```python
from build123d import *

# Parameters (mm, degrees)
CHAFL_N4_SIZE              = 0.2
CHAFL_N5_SIZE              = 0.25
CHAFL_N5_SIZE2             = 0.433012702
CORTAR_EXTRUIR2_DEPTH      = 17.552945357
CORTAR_EXTRUIR2_DEPTH_BACK = 17.552945357
CROQUIS4_W                 = 0.8
CROQUIS4_H                 = 6


with BuildPart() as part:
    # Croquis3 → Revolución1 (revolve)
    with BuildSketch(Plane.XY, mode=Mode.PRIVATE) as revoluci_n1_sk:
        Polygon((-1.6, 0), (-1.6, 16), (-2.4, 16), (-2.4, 13), (-3, 13), (-3, 7.5), (-2.1, 7.5), (-2.1, 5.5), (-3, 5.5), (-3, 0), align=None)
    revolve(revoluci_n1_sk.sketch.rotate(Axis((0, 0, 0), (0, 1, 0)), 270), axis=Axis((0, 0, 0), (0, 1, 0)))

    # Chaflán4
    chafl_n4_edges = [part.edges().sort_by_distance(p)[0] for p in [
        (0, 16, 2.4),
        (0, 0, 3),
    ]]
    chamfer(chafl_n4_edges, length=CHAFL_N4_SIZE)

    # Chaflán5
    chafl_n5_edges = [part.edges().sort_by_distance(p)[0] for p in [
        (0, 16, 1.6),
    ]]
    chafl_n5_side = [part.faces().sort_by_distance(p)[0] for p in [
        (0, 16, 2.137774603),
    ]]
    chamfer(chafl_n5_edges, length=CHAFL_N5_SIZE, length2=CHAFL_N5_SIZE2, reference=chafl_n5_side[0])

    # Croquis4 → Cortar-Extruir2 (cut, two sides: drawn at the far end of the back side and taken through both)
    with BuildSketch(Plane.XY.offset(-CORTAR_EXTRUIR2_DEPTH_BACK)):
        with Locations((-2.6, 6.5)):
            Rectangle(CROQUIS4_W, CROQUIS4_H)
        with Locations((2.6, 6.5)):
            Rectangle(CROQUIS4_W, CROQUIS4_H)
    extrude(amount=CORTAR_EXTRUIR2_DEPTH + CORTAR_EXTRUIR2_DEPTH_BACK, mode=Mode.SUBTRACT)


solid = part.part
```
Here's how the part is built. I have some questions about the finished solid (model axes, mm). A direction names the side the tool comes from. Give positions to 0.01 mm unless a question says otherwise; leave off trailing zeros. Write each loop counter-clockwise with the first axis right and the second up, starting at its lowest first coordinate (ties: lowest second). Pieces come first, ordered by that corner, then holes. Notation, with made-up numbers: M 62.25,-33 L 91.25,-33 A22 cw 91.25,-18 Z; hole C 23.25,-30.75 d6. An arc over 180 degrees is marked long. Put each result on its own line as item: value. Start each with the question number.
Item 1: I need wall thicknesses on L1, parallel to Z at x = -0.1, y = 8; L2, parallel to X at y = 8, z = 0. Which ranges of each line are inside material? Lowest first, please. Write a range as from..to.
Item 2: Will these pins go through, and if not, where does the flat tip stop? pin 1 (2 mm diameter, centred on y = 8, z = 0, fed in from +X); pin 2 (1.3 mm diameter, centred on x = 0, z = 0.5, fed in from -Y).
Item 3: On a 3-axis mill with a long thin cutter (end or side, diameter ignored), from which of +Z, -Z, +X, -X, +Y, -Y can I reach the whole of each face in a straight line? I mean faces 4 (the flat face through (2.5, 3.5, 0)), 5 (the cylindrical face through (-0.631, 6.486, -2.003)), 6 (the flat face through (-2.2, 8, 0)). Say none if no direction works.
Item 4: If we section it at C-C, the plane y = 4.75: Write out the boundary of the cut face in (x, z), then the cut area to 3 significant figures.
Item 5: If we section it at B-B, the plane x = 0: Write out the boundary of the cut face in (y, z), then the cut area to 3 significant figures.
Item 6: Thinking about a two-plate mould opening in Z: for faces 1 (the flat face through (-2.2, 4, 0)), 2 (the cylindrical face through (0.97, 7.89, 1.27)), 3 (the cylindrical face through (-2.024, 14.38, -1.29)), which applies, +Z half, -Z half, draft (parallel to the pull), parting line (faces both ways), or undercut?
Item 7: If we section it at D-D, the plane y = 14.5: Write out the boundary of the cut face in (x, z), then the cut area to 3 significant figures.
Values:
1. L1: -3..-1.6, 1.6..3
1. L2: -2.2..-1.6, 1.6..2.2
2. pin 1: x = 2.2
2. pin 2: through
3. face 4: +Z, -Z, +X
3. face 5: none
3. face 6: +Z, -Z, -X
4. outline: M -2.2,-2.04 A3 ccw 2.2,-2.04 L 2.2,2.04 A3 ccw -2.2,2.04 Z; hole C 0,0 d3.2
4. area: 15.7 mm²
5. outline: M 0,-2.8 L 0.2,-3 L 5.5,-3 L 5.5,-2.1 L 7.5,-2.1 L 7.5,-3 L 13,-3 L 13,-2.4 L 15.8,-2.4 L 16,-2.2 L 16,-1.85 L 15.57,-1.6 L 0,-1.6 Z; M 0,1.6 L 15.57,1.6 L 16,1.85 L 16,2.2 L 15.8,2.4 L 13,2.4 L 13,3 L 7.5,3 L 7.5,2.1 L 5.5,2.1 L 5.5,3 L 0.2,3 L 0,2.8 Z
5. area: 37.4 mm²
6. face 1: draft
6. face 2: undercut
6. face 3: parting line
7. outline: C 0,0 d4.8; hole C 0,0 d3.2
7. area: 10.1 mm²
